```python
from build123d import *

# Parameters (mm, degrees)
SKETCH_1_W          = 270
SKETCH_1_H          = 175
EXTRUDE_1_DEPTH     = 15
SKETCH_2_W          = 20
SKETCH_2_H          = 20
EXTRUDE_5_DEPTH     = 275
SKETCH_5_W          = 110
SKETCH_5_H          = 20
SKETCH_5_W_2        = 20
SKETCH_5_H_2        = 105
EXTRUDE_6_DEPTH     = 10
SKETCH_6_W          = 110
SKETCH_6_H          = 20
SKETCH_6_W_2        = 20
SKETCH_6_H_2        = 105
EXTRUDE_7_DEPTH     = 10
SKETCH_7_W          = 270
SKETCH_7_H          = 15
EXTRUDE_8_DEPTH     = 5
SKETCH_8_W          = 270
SKETCH_8_H          = 5
CUT_EXTRUDE_1_DEPTH = 2
SKETCH_10_W         = 270
SKETCH_10_H         = 10
CUT_EXTRUDE_2_DEPTH = 3


with BuildPart() as part:
    # Sketch 1 → Extrude 1 (new body)
    with BuildSketch(Plane(origin=(0, 0, 0), x_dir=(1, 0, 0), z_dir=(0, 1, 0))):
        Rectangle(SKETCH_1_W, SKETCH_1_H)
    extrude(amount=EXTRUDE_1_DEPTH)

    # Sketch 2 → Extrude 5 (add)
    with BuildSketch(Plane.XZ):
        with Locations((65, -62.5)):
            Rectangle(SKETCH_2_W, SKETCH_2_H)
        with Locations((65, 62.5)):
            Rectangle(SKETCH_2_W, SKETCH_2_H)
        with Locations((-65, 62.5)):
            Rectangle(SKETCH_2_W, SKETCH_2_H)
        with Locations((-65, -62.5)):
            Rectangle(SKETCH_2_W, SKETCH_2_H)
    extrude(amount=EXTRUDE_5_DEPTH)

    # Sketch 5 → Extrude 6 (add)
    with BuildSketch(Plane.XZ):
        with Locations((0, 62.5)):
            Rectangle(SKETCH_5_W, SKETCH_5_H)
        with Locations((-65, 0)):
            Rectangle(SKETCH_5_W_2, SKETCH_5_H_2)
        with Locations((0, -62.5)):
            Rectangle(SKETCH_5_W, SKETCH_5_H)
        with Locations((65, 0)):
            Rectangle(SKETCH_5_W_2, SKETCH_5_H_2)
    extrude(amount=EXTRUDE_6_DEPTH)

    # Sketch 6 → Extrude 7 (add)
    with BuildSketch(Plane(origin=(0, -265, 0), x_dir=(-1, 0, 0), z_dir=(0, -1, 0))):
        with Locations((0, -62.5)):
            Rectangle(SKETCH_6_W, SKETCH_6_H)
        with Locations((65, 0)):
            Rectangle(SKETCH_6_W_2, SKETCH_6_H_2)
        with Locations((0, 62.5)):
            Rectangle(SKETCH_6_W, SKETCH_6_H)
        with Locations((-65, 0)):
            Rectangle(SKETCH_6_W_2, SKETCH_6_H_2)
    extrude(amount=EXTRUDE_7_DEPTH)

    # Sketch 7 → Extrude 8 (add)
    with BuildSketch(Plane(origin=(0, 15, 0), x_dir=(1, 0, 0), z_dir=(0, 1, 0))):
        with Locations((0, 60)):
            Rectangle(SKETCH_7_W, SKETCH_7_H)
        with Locations((0, -60)):
            Rectangle(SKETCH_7_W, SKETCH_7_H)
    extrude(amount=EXTRUDE_8_DEPTH)

    # Sketch 8 → Cut-Extrude 1 (cut)
    with BuildSketch(Plane(origin=(0, 20, 0), x_dir=(1, 0, 0), z_dir=(0, 1, 0))):
        with Locations((0, -60)):
            Rectangle(SKETCH_8_W, SKETCH_8_H)
        with Locations((0, 60)):
            Rectangle(SKETCH_8_W, SKETCH_8_H)
    extrude(amount=-CUT_EXTRUDE_1_DEPTH, mode=Mode.SUBTRACT)

    # Sketch 10 → Cut-Extrude 2 (cut)
    with BuildSketch(Plane(origin=(0, 18, 0), x_dir=(1, 0, 0), z_dir=(0, 1, 0))):
        with Locations((0, -60)):
            Rectangle(SKETCH_10_W, SKETCH_10_H)
        with Locations((0, 60)):
            Rectangle(SKETCH_10_W, SKETCH_10_H)
    extrude(amount=-CUT_EXTRUDE_2_DEPTH, mode=Mode.SUBTRACT)


solid = part.part
```
Could you check a few things on this model? Use its own coordinates, in mm. A direction names the side the tool comes from. Round coordinates to 2 decimals unless told otherwise and drop trailing zeros. Loops run counter-clockwise (first coordinate to the right, second up) from the corner with the lowest first, then second, coordinate; pieces in that order, holes last. Notation, with made-up numbers: (16, 40.25) -> (56, 40.25) arc R21 ccw to (56, 69.25) -> close; hole circle Ø5 at (83, -20). An arc over 180 degrees is marked (long way). Put each result on its own line as item: value.
Q1. I want a section at D-D on x = -109.5. Write out the boundary of the cut face in (y, z).
Checks:
outline: (0, -87.5) -> (15, -87.5) -> (15, -67.5) -> (20, -67.5) -> (20, -62.5) -> (18, -62.5) -> (18, -65) -> (15, -65) -> (15, -55) -> (18, -55) -> (18, -57.5) -> (20, -57.5) -> (20, -52.5) -> (15, -52.5) -> (15, 52.5) -> (20, 52.5) -> (20, 57.5) -> (18, 57.5) -> (18, 55) -> (15, 55) -> (15, 65) -> (18, 65) -> (18, 62.5) -> (20, 62.5) -> (20, 67.5) -> (15, 67.5) -> (15, 87.5) -> (0, 87.5) -> close
Q2. Please list where these lines run through material, in increasing order: line 1 (X direction, y = -167, z = -61.5); line 2 (Y direction, x = -53.5, z = 22); line 3 (Z direction, x = 62.5, y = -208.5). Write a range as from..to.
Checks:
line 1: -75..-55, 55..75
line 2: 0..15
line 3: -72.5..-52.5, 52.5..72.5
Q3. I want a section at A-A on z = 18.5. Write out the boundary of the cut face in (x, y), and give its area (3 significant figures).
Checks:
outline: (-135, 0) -> (-75, 0) -> (-75, -10) -> (-55, -10) -> (-55, 0) -> (55, 0) -> (55, -10) -> (75, -10) -> (75, 0) -> (135, 0) -> (135, 15) -> (-135, 15) -> close; (-75, -275) -> (-55, -275) -> (-55, -265) -> (-75, -265) -> close; (55, -275) -> (75, -275) -> (75, -265) -> (55, -265) -> close
area: 4,850 mm2
Q4. I want a section at B-B on y = -5. Write out the boundary of the cut face in (x, z).
Checks:
outline: (-75, -72.5) -> (75, -72.5) -> (75, 72.5) -> (-75, 72.5) -> close; hole (-55, -52.5) -> (55, -52.5) -> (55, 52.5) -> (-55, 52.5) -> close
Q5. Thinking about a two-plate mould opening in Y: for faces 1 (the flat face through (-65, -136, 52.5)), 2 (the flat face through (-55, -5, -1)), 3 (the flat face through (-1, 0, -1)), which applies, pulls with the +Y half, pulls with the -Y half, needs draft (parallel to the pull), parting line crosses it, or undercut?
Checks:
face 1: undercut
face 2: needs draft
face 3: pulls with the -Y half
Q6. Which directions (+Z, -Z, +X, -X, +Y, -Y) give clear straight access to the entire face, cutting with the end or side of a thin tool? Please do faces 4 (the flat face through (-55, -136, 62)), 5 (the flat face through (-75, -147, -54)), 6 (the flat face through (-2, 15, -78)), 7 (the flat face through (56, -147, 72.5)), 8 (the flat face through (65, -136, -52.5)).
Checks:
face 4: +Z, -Z
face 5: +Z, -Z, -X, -Y
face 6: -Z, +X, -X, +Y
face 7: +Z, +X, -X, -Y
face 8: +X, -X
Q7. I want a section at C-C on y = -160. Write out the boundary of the cut face in (x, z), and give its area (3 significant figures).
Checks:
outline: (-75, -72.5) -> (-55, -72.5) -> (-55, -52.5) -> (-75, -52.5) -> close; (-75, 52.5) -> (-55, 52.5) -> (-55, 72.5) -> (-75, 72.5) -> close; (55, -72.5) -> (75, -72.5) -> (75, -52.5) -> (55, -52.5) -> close; (55, 52.5) -> (75, 52.5) -> (75, 72.5) -> (55, 72.5) -> close
area: 1,600 mm2
Q8. For pin 1 Ø1 at (x, y) = (68, -69) entering from +Z; pin 2 Ø16 at (y, z) = (-138, -63.5) entering from +X; pin 3 Ø8 at (x, z) = (-17.5, -36.5) entering from -Y; pin 4 Ø5 at (x, z) = (2.5, -59) entering from +Y, each with a flat end and sliding along its axis, tell me the tip position at first contact or that it passes through.
Checks:
pin 1: z = 72.5
pin 2: x = 75
pin 3: y = 0
pin 4: y = 20
